Autodesk Inventor part; units mm, degrees
ref_plane "YZ Plane" through (0, 0, 0) normal (1, 0, 0) x (0, 1, 0)
ref_plane "XZ Plane" through (0, 0, 0) normal (0, 1, 0) x (-1, 0, 0)
ref_plane "XY Plane" through (0, 0, 0) normal (0, 0, 1) x (1, 0, 0)
sketch "Sketch1" plane through (0, 0, 0) normal (0, 0, 1) x (1, 0, 0)
  line L0 (0, 0) -> (20, 0)
  line L1 (20, 0) -> (20, 20)
  line L2 (20, 20) -> (0, 20)
  line L3 (0, 20) -> (0, 0)
  dimension "d0" = 20
  dimension "d1" = 20
extrude "Extrusion1" add sketch "Sketch1" along normal blind 5
sketch "Sketch2" plane through (0, 0, 5) normal (0, 0, 1) x (1, 0, 0)
  line L0 (0, 0) -> (10, 0)
  line L1 (0, 0) -> (20, 0)
  line L2 (10, 0) -> (10, 10)
  circle A0 centre (10, 10) radius 8
  dimension "d4" = 10
  dimension "d5" = 10
  dimension "d6" = 16
extrude "Extrusion2" cut sketch "Sketch2" against normal through all
thread "Thread1"
properties part number "DC MOTOR NUT FOR CAPPING SYSTEM"
The listing builds one solid part. Answer for the finished solid, in the listing's coordinates (mm). Round coordinates to 2 decimals unless told otherwise and drop trailing zeros. Loops run counter-clockwise (first coordinate to the right, second up) from the corner with the lowest first, then second, coordinate; pieces in that order, holes last.
1) For a pull along Y with two mould halves and no side action, classify faces 1 (the face through (8.27, 2.19, 2.54)), 2 (the face through (10, 20, 2)), 3 (the face through (5, 17, 0)) as released by +Y, released by -Y, zero draft, split by the parting line, or undercut.
Outcome:
face 1: undercut
face 2: released by +Y
face 3: zero draft
2) Consider line 1 (Y direction, x = 10, z = 0.75); line 2 (Y direction, x = 17.25, z = 0.75). Determine where each line is inside the solid, lowest interval first.
Outcome:
line 1: y = 0 to 2, 18 to 20
line 2: y = 0 to 6.62, 13.38 to 20
3) A cutting plane is placed at C-C on z = 2.95. Determine the outline of the cut face in (x, y), plus the area to 3 significant figures.
Outcome:
outline: (0, 0) - (20, 0) - (20, 20) - (0, 20) - close; hole circle Ø16 at (10, 10)
area: 199 mm2
4) A cutting plane is placed at A-A on y = 10. Determine the outline of the cut face in (x, z), plus the area to 3 significant figures.
Outcome:
outline: (0, 0) - (2, 0) - (2, 5) - (0, 5) - close; (18, 0) - (20, 0) - (20, 5) - (18, 5) - close
area: 20.0 mm2
